Design review of the part shown in the three views and the two pictorial views. Dimensions are in mm from the part's minimum x, y and z. A direction names the side the tool comes from. Coordinates: 2 decimals unless noted, no trailing zeros. Order: outer loops, then holes, each group sorted by start corner. A loop starts at its lowest first (then second) coordinate and runs counter-clockwise, first axis right, second up. Notation, with made-up numbers: (-13, 89.25) -> (44, 89.25) arc R29 ccw to (44, 114.25) -> close; hole circle Ø9 at (63, 62). An arc over 180 degrees is marked (long way). Write item = value, one per line. Start each with the question number.
1) Insertion check: pin 1 Ø2.5 at (x, z) = (26.985, 16) entering from +Y; pin 2 Ø14.5 at (y, z) = (37, 80.5) entering from +X (3 decimals); pin 3 Ø12 at (x, z) = (12.5, 41) entering from -Y; pin 4 Ø3.5 at (x, z) = (26.985, 6) entering from +Y (3 decimals). Each pin has a flat end and moves straight along its axis. Give the tip position at first contact, or say it passes through.
2) Machinability: for the marked faces 1 and 2, which of the approach directions +Z, -Z, +X, -X, +Y, -Y give a long, thin tool a straight path to every point of the face, cutting with its end or side? Answer none if there is none.
3) Consider section A-A on z = 29.9. Give the boundary of the cut face in (x, y) (3 decimals).
4) Consider section C-C on z = 16. Give the boundary of the cut face in (x, y) (3 decimals).
5) Consider section B-B on x = 40.8. Give the boundary of the cut face in (y, z) (3 decimals).
6) Consider section D-D on y = 10. Give the boundary of the cut face in (x, z) (3 decimals).
7) Wall thickness on probe 1 along X at (y, z) = (1.8, 110.1); probe 2 along Z at (x, y) = (40.8, 1.9); probe 3 along Z at (x, y) = (40, 1): over which ranges is each line inside the solid? List them lowest first. Write a range as [from, to].
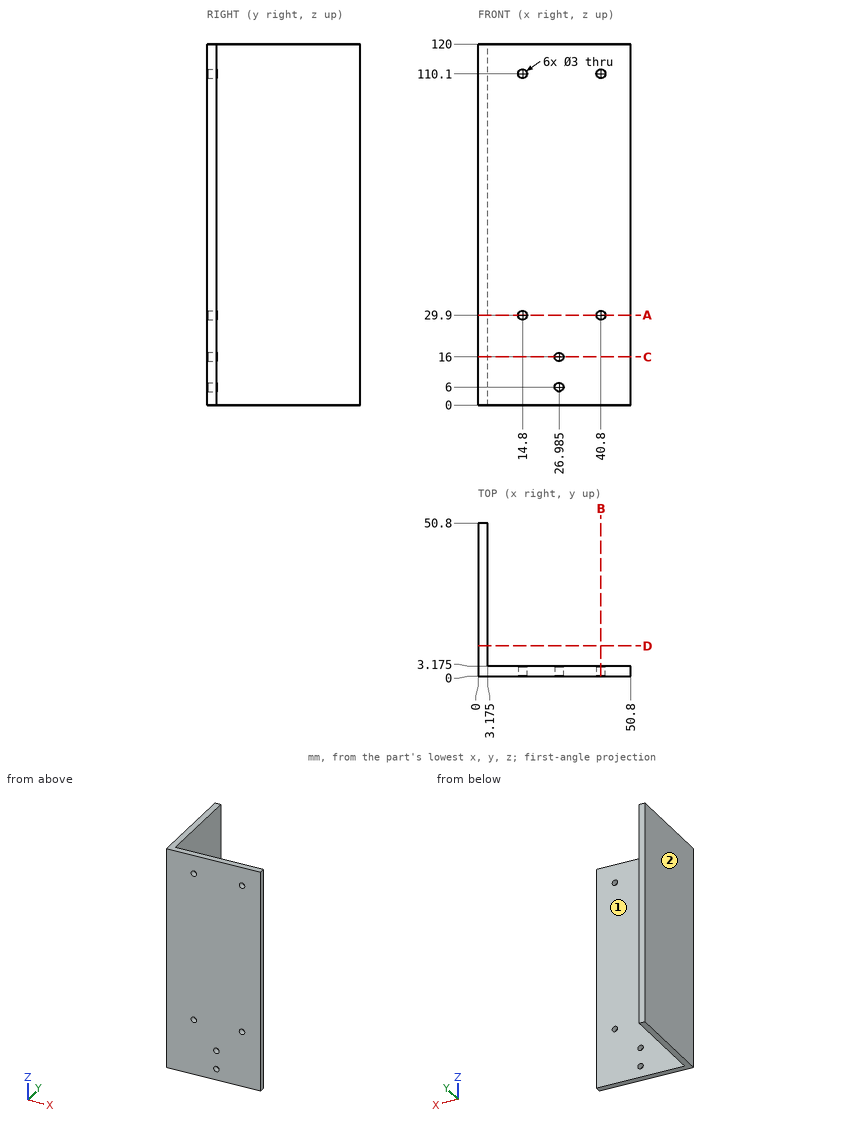
Answer sheet:
q1.pin_1 = through
q1.pin_2 = 3.175
q1.pin_3 = 0
q1.pin_4 = 3.175
q2.face_1 = +Z, -Z, +X, +Y
q2.face_2 = +Z, -Z, -X, +Y, -Y
q3.outline = (0, 0) -> (13.3, 0) -> (13.3, 3.175) -> (3.175, 3.175) -> (3.175, 50.8) -> (0, 50.8) -> close; (16.3, 0) -> (39.3, 0) -> (39.3, 3.175) -> (16.3, 3.175) -> close; (42.3, 0) -> (50.8, 0) -> (50.8, 3.175) -> (42.3, 3.175) -> close
q4.outline = (0, 0) -> (25.485, 0) -> (25.485, 3.175) -> (3.175, 3.175) -> (3.175, 50.8) -> (0, 50.8) -> close; (28.485, 0) -> (50.8, 0) -> (50.8, 3.175) -> (28.485, 3.175) -> close
q5.outline = (0, 0) -> (3.175, 0) -> (3.175, 28.4) -> (0, 28.4) -> close; (0, 31.4) -> (3.175, 31.4) -> (3.175, 108.6) -> (0, 108.6) -> close; (0, 111.6) -> (3.175, 111.6) -> (3.175, 120) -> (0, 120) -> close
q6.outline = (0, 0) -> (3.175, 0) -> (3.175, 120) -> (0, 120) -> close
q7.probe_1 = [0, 13.3], [16.3, 39.3], [42.3, 50.8]
q7.probe_2 = [0, 28.4], [31.4, 108.6], [111.6, 120]
q7.probe_3 = [0, 28.63], [31.17, 108.83], [111.37, 120]
